```python
from build123d import *

# Parameters (mm, degrees)
BOSS_EXTRUDE1_DEPTH      = 53.65
BOSS_EXTRUDE1_DEPTH_BACK = 53.65
CUT_EXTRUDE1_DEPTH       = 50
CUT_EXTRUDE2_DEPTH       = 40
CUT_EXTRUDE2_DEPTH_BACK  = 40
SKETCH4_W                = 8
SKETCH4_H                = 19.5
BOSS_EXTRUDE2_DEPTH      = 1.5
SKETCH5_W                = 16.8
SKETCH5_H                = 20.35
BOSS_EXTRUDE3_DEPTH      = 1.5
CUT_EXTRUDE3_DEPTH       = 30
CUT_EXTRUDE3_DEPTH_BACK  = 30
CUT_EXTRUDE4_DEPTH       = 30
SKETCH8_R                = 2.15
CUT_EXTRUDE5_DEPTH       = 30
CUT_EXTRUDE6_DEPTH       = 10.8
CUT_EXTRUDE7_DEPTH       = 10.8
SKETCH13_W               = 20
SKETCH13_H               = 1.715
CUT_EXTRUDE8_DEPTH       = 5
CUT_EXTRUDE8_DEPTH_BACK  = 5
CUT_EXTRUDE9_DEPTH       = 0.6
SKETCH16_W               = 12
SKETCH16_H               = 2.5
CUT_EXTRUDE10_DEPTH      = 3.5


with BuildPart() as part:
    # Sketch1 → Boss-Extrude1 (new body, two sides)
    with BuildSketch(Plane.XY) as boss_extrude1_sk:
        with BuildLine():
            Line((-5, 1.3), (20, 1.3))
            Line((20, 1.3), (20, 10.3))
            ThreePointArc((20, 10.3), (19.853553391, 10.653553391), (19.5, 10.8))
            Line((19.5, 10.8), (7.5, 10.8))
            ThreePointArc((7.5, 10.8), (7.146446609, 10.946446609), (7, 11.3))
            Line((7, 11.3), (7, 30.113329403))
            ThreePointArc((7, 30.113329403), (6.679537553, 32.531612644), (6.067046966, 34.89289308))
            ThreePointArc((6.067046966, 34.89289308), (5.958046762, 35.042763181), (5.781791158, 35.1))
            Line((5.781791158, 35.1), (-5, 35.1))
            Line((-5, 35.1), (-5, 1.3))
        make_face()
    extrude(amount=BOSS_EXTRUDE1_DEPTH)
    extrude(boss_extrude1_sk.sketch, amount=-BOSS_EXTRUDE1_DEPTH_BACK)

    # Sketch2 → Cut-Extrude1 (cut)
    with BuildSketch(Plane(origin=(0, 0, 0), x_dir=(1, 0, 0), z_dir=(0, 1, 0))):
        with BuildLine():
            Line((-50, 53.65), (-50, -53.65))
            Line((-50, -53.65), (0, -53.65))
            Line((0, -53.65), (0, -22.228541033))
            ThreePointArc((0, -22.228541033), (-1.117187677, -20.892122365), (-0.57947873, -19.235320551))
            Line((-0.57947873, -19.235320551), (0.516087478, -18.210754943))
            ThreePointArc((0.516087478, -18.210754943), (1.125563929, -16.438315605), (0, -14.939613301))
            Line((0, -14.939613301), (0, 53.65))
            Line((0, 53.65), (-50, 53.65))
        make_face()
    extrude(amount=CUT_EXTRUDE1_DEPTH, mode=Mode.SUBTRACT)

    # Sketch3 → Cut-Extrude2 (cut, two sides)
    with BuildSketch(Plane(origin=(0, 0, 0), x_dir=(0, 0, -1), z_dir=(1, 0, 0))) as cut_extrude2_sk:
        Polygon((-26, 2.9), (-26, -8.174443219), (14, -7.963716906), (14, 2.543524479), (16.45, 3.2), (16.45, 4.4), (-19.05, 4.4), (-19.05, 2.9), align=None)
    extrude(amount=CUT_EXTRUDE2_DEPTH, mode=Mode.SUBTRACT)
    extrude(cut_extrude2_sk.sketch, amount=-CUT_EXTRUDE2_DEPTH_BACK, mode=Mode.SUBTRACT)

    # Sketch4 → Boss-Extrude2 (add)
    with BuildSketch(Plane(origin=(0, 0, 0), x_dir=(1, 0, 0), z_dir=(0, 1, 0))):
        with Locations((12.8, 25.75)):
            Rectangle(SKETCH4_W, SKETCH4_H)
    extrude(amount=BOSS_EXTRUDE2_DEPTH)

    # Sketch5 → Boss-Extrude3 (add)
    with BuildSketch(Plane(origin=(0, 0, 0), x_dir=(1, 0, 0), z_dir=(0, 1, 0))):
        with Locations((8.4, -39.675)):
            Rectangle(SKETCH5_W, SKETCH5_H)
    extrude(amount=BOSS_EXTRUDE3_DEPTH)

    # Sketch6 → Cut-Extrude3 (cut, two sides)
    with BuildSketch(Plane(origin=(0, 0, 0), x_dir=(1, 0, 0), z_dir=(0, 1, 0))) as cut_extrude3_sk:
        with BuildLine():
            Line((13.7, 26.9), (15.2, 26.9))
            ThreePointArc((15.2, 26.9), (18.5, 30.2), (15.2, 33.5))
            Line((15.2, 33.5), (13.7, 33.5))
            ThreePointArc((13.7, 33.5), (10.4, 30.2), (13.7, 26.9))
        make_face()
    extrude(amount=CUT_EXTRUDE3_DEPTH, mode=Mode.SUBTRACT)
    extrude(cut_extrude3_sk.sketch, amount=-CUT_EXTRUDE3_DEPTH_BACK, mode=Mode.SUBTRACT)

    # Sketch7 → Cut-Extrude4 (cut)
    with BuildSketch(Plane(origin=(0, 0, 0), x_dir=(1, 0, 0), z_dir=(0, 1, 0))):
        with BuildLine():
            Line((13, 17.95), (14, 17.95))
            ThreePointArc((14, 17.95), (16.2, 20.15), (14, 22.35))
            Line((14, 22.35), (13, 22.35))
            ThreePointArc((13, 22.35), (10.8, 20.15), (13, 17.95))
        make_face()
    extrude(amount=CUT_EXTRUDE4_DEPTH, mode=Mode.SUBTRACT)

    # Sketch8 → Cut-Extrude5 (cut)
    with BuildSketch(Plane(origin=(0, 0, 0), x_dir=(1, 0, 0), z_dir=(0, 1, 0))):
        with Locations((12.7, -23.05)):
            Circle(SKETCH8_R)
    extrude(amount=CUT_EXTRUDE5_DEPTH, mode=Mode.SUBTRACT)

    # Sketch9 → Cut-Extrude6 (cut)
    with BuildSketch(Plane(origin=(0, 0, 0), x_dir=(1, 0, 0), z_dir=(0, 1, 0))):
        with BuildLine():
            Line((13.7, -38.1), (15.2, -38.1))
            ThreePointArc((15.2, -38.1), (18.5, -34.8), (15.2, -31.5))
            Line((15.2, -31.5), (13.7, -31.5))
            ThreePointArc((13.7, -31.5), (10.4, -34.8), (13.7, -38.1))
        make_face()
    extrude(amount=CUT_EXTRUDE6_DEPTH, mode=Mode.SUBTRACT)

    # Sketch10 → Cut-Extrude7 (cut)
    with BuildSketch(Plane(origin=(0, 0, 0), x_dir=(1, 0, 0), z_dir=(0, 1, 0))):
        with BuildLine():
            Line((13, -48.35), (14, -48.35))
            ThreePointArc((14, -48.35), (16.2, -46.15), (14, -43.95))
            Line((14, -43.95), (13, -43.95))
            ThreePointArc((13, -43.95), (10.8, -46.15), (13, -48.35))
        make_face()
    extrude(amount=CUT_EXTRUDE7_DEPTH, mode=Mode.SUBTRACT)

    # Sketch11 → Cut-Revolve1 (revolve, cut)
    with BuildSketch(Plane(origin=(0, 11.8, 0), x_dir=(1, 0, 0), z_dir=(0, 1, 0))):
        Polygon((0, 10.45), (0, 12.2), (2, 12.2), (2, 13.45), (20, 13.45), (20, 10.45), align=None)
    revolve(axis=Axis((20, 11.8, -10.45), (-1, 0, 0)), mode=Mode.SUBTRACT)

    # Sketch12 → Cut-Revolve2 (revolve, cut)
    with BuildSketch(Plane(origin=(0, 4.8, 0), x_dir=(1, 0, 0), z_dir=(0, 1, 0))):
        Polygon((0, -33.85), (0, -32.1), (2, -32.1), (2, -30.85), (20, -30.85), (20, -33.85), align=None)
    revolve(axis=Axis((20, 4.8, 33.85), (-1, 0, 0)), mode=Mode.SUBTRACT)

    # Sketch13 → Cut-Revolve3 (revolve, cut)
    with BuildSketch(Plane(origin=(0, 31.1, 0), x_dir=(1, 0, 0), z_dir=(0, 1, 0))):
        with Locations((10, -48.4625)):
            Rectangle(SKETCH13_W, SKETCH13_H)
    revolve(axis=Axis((20, 31.1, 49.32), (-1, 0, 0)), mode=Mode.SUBTRACT)

    # Sketch14 → Cut-Extrude8 (cut, two sides)
    with BuildSketch(Plane(origin=(7, 0, 0), x_dir=(0, 0, -1), z_dir=(1, 0, 0))) as cut_extrude8_sk:
        with BuildLine():
            Line((-54.15, 28.1), (-49.15, 28.1))
            ThreePointArc((-49.15, 28.1), (-46.15, 31.1), (-49.15, 34.1))
            Line((-49.15, 34.1), (-54.15, 34.1))
            Line((-54.15, 34.1), (-54.15, 28.1))
        make_face()
    extrude(amount=CUT_EXTRUDE8_DEPTH, mode=Mode.SUBTRACT)
    extrude(cut_extrude8_sk.sketch, amount=-CUT_EXTRUDE8_DEPTH_BACK, mode=Mode.SUBTRACT)

    # Sketch15 → Cut-Extrude9 (cut)
    with BuildSketch(Plane(origin=(0, 10.8, 0), x_dir=(1, 0, 0), z_dir=(0, 1, 0))):
        with BuildLine():
            Line((12.7, -27.6), (20, -27.6))
            Line((20, -27.6), (20, -18.5))
            Line((20, -18.5), (12.7, -18.5))
            ThreePointArc((12.7, -18.5), (8.15, -23.05), (12.7, -27.6))
        make_face()
    extrude(amount=-CUT_EXTRUDE9_DEPTH, mode=Mode.SUBTRACT)

    # Sketch16 → Cut-Extrude10 (cut)
    with BuildSketch(Plane(origin=(0, 0, 0), x_dir=(1, 0, 0), z_dir=(0, 1, 0))):
        with Locations((9.65, 15.2)):
            Rectangle(SKETCH16_W, SKETCH16_H)
    extrude(amount=CUT_EXTRUDE10_DEPTH, mode=Mode.SUBTRACT)


solid = part.part
```
The model under review builds one solid part; all positions refer to its coordinate system, in mm. A direction names the side the tool comes from. Round coordinates to 2 decimals unless told otherwise and drop trailing zeros. Loops run counter-clockwise (first coordinate to the right, second up) from the corner with the lowest first, then second, coordinate; pieces in that order, holes last.
Item 1: Take a section at C-C (x = 11.75). Give the number of separate pieces and of enclosed holes in the cut face, then the cut area to 3 significant figures.
Determined:
separate pieces: 6
enclosed holes: 0
area: 710 mm2
Item 2: For line 1 (Y direction, x = 0.65, z = 33.85); line 2 (Y direction, x = 1.35, z = 49.32) (3 decimals); line 3 (Y direction, x = 19, z = -41), list the stretches that pass through material, from the lowest coordinate up.
Determined:
line 1: y = 0 to 3.05, 6.55 to 35.1
line 2: y = 0 to 29.385, 32.815 to 35.1
line 3: y = 1.3 to 10.8
Item 3: Clearance check with flat-ended pins moving along their axes: pin 1 Ø1.4 at (y, z) = (0.5, -24) entering from -X; pin 2 Ø1 at (x, z) = (2.5, -33.5) entering from -Y; pin 3 Ø1 at (x, z) = (8, 17) entering from -Y. State where each tip first meets the part, or that it passes through.
Determined:
pin 1: stops at x = 8.8
pin 2: stops at y = 1.3
pin 3: stops at y = 4.4
Item 4: Take a section at B-B (y = 26). Write out the cut boundary in (x, z).
Determined:
outline: (-0.58, 19.24) - (0.52, 18.21) arc R2 cw to (0, 14.94) - (0, -53.65) - (7, -53.65) - (7, 53.65) - (0, 53.65) - (0, 22.23) arc R1.8 ccw to start
Item 5: For faces 5 (the face through (1.799, 2.867, -15.208)), 6 (the face through (8.15, 10.5, 22.95)), 7 (the face through (4, 34.1, 51)), 8 (the face through (9.13, 5.95, 31.08)), 9 (the face through (10.8, 5.3, 46.1)), list the 3-axis set-ups (+Z, -Z, +X, -X, +Y, -Y) from which the entire face can be reached by the end or side of a thin tool; tool diameter is ignored.
Determined:
face 5: +X, -X
face 6: +X, +Y
face 7: +Z, +X
face 8: +X
face 9: +Y, -Y
Item 6: Take a section at A-A (z = 10). Write out the cut boundary in (x, y).
Determined:
outline: (0, 4.4) - (20, 4.4) - (20, 10.3) arc R0.5 ccw to (19.5, 10.8) - (7.5, 10.8) arc R0.5 cw to (7, 11.3) - (7, 30.11) arc R20 ccw to (6.07, 34.89) arc R0.3 ccw to (5.78, 35.1) - (0, 35.1) - close
Item 7: Mouldability with a two-part tool opening along X and no side actions: class faces 1 (the face through (16.2, 5.3, 46.2)), 2 (the face through (11, 10.8, -33)), 3 (the face through (10.8, 5.3, -20.2)), 4 (the face through (0, 18, -19)) as released by +X, released by -X, zero draft, split by the parting line, or undercut.
Determined:
face 1: undercut
face 2: zero draft
face 3: undercut
face 4: released by -X
